Read the model definition and answer for the solid it produces. Units are mm, in the model's axes. Face numbers are marked on the shaded views. A direction names the side the tool comes from. Coordinates: 2 decimals unless noted, no trailing zeros. Order: outer loops, then holes, each group sorted by start corner. A loop starts at its lowest first (then second) coordinate and runs counter-clockwise, first axis right, second up. Notation, with made-up numbers: (19, -28) -> (30, -28) arc R13 ccw to (30, -8) -> close; hole circle Ø1 at (-24.75, 0.5). An arc over 180 degrees is marked (long way). Return JSON: item names as keys, results as strings. Group by question number.
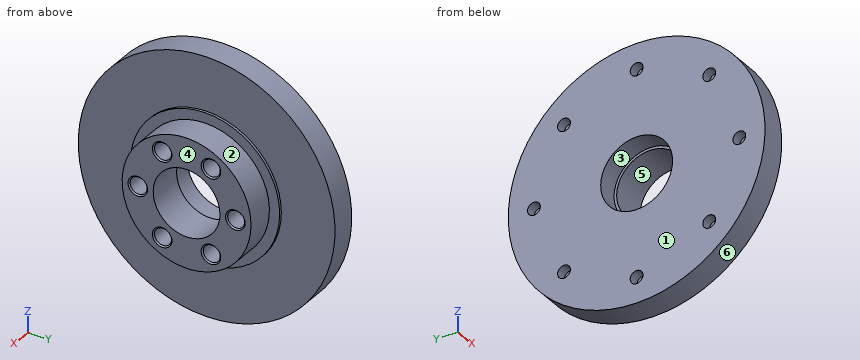
```python
from build123d import *

# Parameters (mm, degrees)
SKETCH3_R          = 2.5
CUT_EXTRUDE1_DEPTH = 4
SKETCH4_R          = 3.3
CUT_EXTRUDE2_DEPTH = 10
CHAMFER1_SIZE      = 0.5


with BuildPart() as part:
    # Sketch2 → Revolve1 (revolve)
    with BuildSketch(Plane.XY, mode=Mode.PRIVATE) as revolve1_sk:
        Polygon((0, 50), (10, 50), (10, 29.1), (11, 29.1), (11, 25.1), (22, 25.1), (22, 13), (8, 13), (8, 14), (0, 14), align=None)
    revolve(revolve1_sk.sketch.rotate(Axis((0, 0, 0), (1, 0, 0)), 90), axis=Axis((0, 0, 0), (1, 0, 0)))

    # Sketch3 → Cut-Extrude1 (cut)
    with BuildSketch(Plane(origin=(0, 0, 0), x_dir=(0, 0, -1), z_dir=(1, 0, 0))):
        with Locations((0, 40)):
            Circle(SKETCH3_R)
        with Locations((28.284271247, 28.284271247)):
            Circle(SKETCH3_R)
        with Locations((40, 0)):
            Circle(SKETCH3_R)
        with Locations((28.284271247, -28.284271247)):
            Circle(SKETCH3_R)
        with Locations((0, -40)):
            Circle(SKETCH3_R)
        with Locations((-28.284271247, -28.284271247)):
            Circle(SKETCH3_R)
        with Locations((-40, 0)):
            Circle(SKETCH3_R)
        with Locations((-28.284271247, 28.284271247)):
            Circle(SKETCH3_R)
    extrude(amount=CUT_EXTRUDE1_DEPTH, mode=Mode.SUBTRACT)

    # Sketch4 → Cut-Extrude2 (cut)
    with BuildSketch(Plane(origin=(22, 0, 0), x_dir=(0, 0, -1), z_dir=(1, 0, 0))):
        with Locations((0, 19)):
            Circle(SKETCH4_R)
        with Locations((16.454482672, 9.5)):
            Circle(SKETCH4_R)
        with Locations((16.454482672, -9.5)):
            Circle(SKETCH4_R)
        with Locations((0, -19)):
            Circle(SKETCH4_R)
        with Locations((-16.454482672, -9.5)):
            Circle(SKETCH4_R)
        with Locations((-16.454482672, 9.5)):
            Circle(SKETCH4_R)
    extrude(amount=-CUT_EXTRUDE2_DEPTH, mode=Mode.SUBTRACT)

    # Chamfer1
    chamfer1_edges = [part.edges().sort_by_distance(p)[0] for p in [
        (22, 19, 3.3),
        (22, 9.5, 19.754482672),
        (22, -9.5, 19.754482672),
        (22, -19, 3.3),
        (22, -9.5, -13.154482672),
        (22, 9.5, -13.154482672),
    ]]
    chamfer(chamfer1_edges, length=CHAMFER1_SIZE)


solid = part.part
```
1. Find section D-D on x = 2. Give the number of separate pieces and of enclosed holes in the cut face, and give its area (3 significant figures).
2. Find section A-A on x = 13.5. Determine the outline of the cut face in (y, z).
3. Which of the six approach directions +Z, -Z, +X, -X, +Y, -Y give full straight-line access (tool end or side, diameter ignored) to the marked faces 1 and 2?
4. Given pin 1 (3 mm diameter, centred on y = 0, z = 40, fed in from -X); pin 2 (8 mm diameter, centred on y = 28.28, z = 28.28, fed in from +X); pin 3 (12 mm diameter, centred on x = 19.5, z = -18, fed in from -Y), each flat-ended and moving along its own axis, determine where each tip first touches the part or whether it passes through.
5. Find section C-C on z = 40. Determine the outline of the cut face in (x, y), and give its area (3 significant figures).
6. Straight lines are drawn through the part: L1, parallel to Y at x = 15, z = 0; L2, parallel to Y at x = 3.05, z = 0; L3, parallel to X at y = 16, z = -38. For each, find the intervals that lie inside material, in ascending order.
7. Find section B-B on y = 0. Determine the outline of the cut face in (x, z), and give its area (3 significant figures).
8. For a pull along Y with two mould halves and no side action, classify the marked faces 3, 4, 5 and 6 as released by +Y, released by -Y, zero draft, split by the parting line, or undercut.
Result:
{
 "1": {"separate pieces": "1", "enclosed holes": "9", "area": "7,080 mm^2"},
 "2": {"outline": "circle Ø50.2 at (0, 0); hole circle Ø6.6 at (-19, 0); hole circle Ø26 at (0, 0); hole circle Ø6.6 at (-9.5, -16.45); hole circle Ø6.6 at (-9.5, 16.45); hole circle Ø6.6 at (9.5, -16.45); hole circle Ø6.6 at (9.5, 16.45); hole circle Ø6.6 at (19, 0)"},
 "3": {"face 1": "+Z, -Z, -X, +Y, -Y", "face 2": "+X"},
 "4": {"pin 1": "x = 4", "pin 2": "x = 10", "pin 3": "y = -22.05"},
 "5": {"outline": "(0, -30) -> (10, -30) -> (10, 30) -> (0, 30) -> (0, 2.5) -> (4, 2.5) -> (4, -2.5) -> (0, -2.5) -> close", "area": "580 mm^2"},
 "6": {"L1": "-25.1 to -22.3, -15.7 to -13, 13 to 15.7, 22.3 to 25.1", "L2": "-50 to -42.5, -37.5 to -14, 14 to 37.5, 42.5 to 50", "L3": "0 to 10"},
 "7": {"outline": "(0, -50) -> (10, -50) -> (10, -29.1) -> (11, -29.1) -> (11, -25.1) -> (22, -25.1) -> (22, -13) -> (8, -13) -> (8, -14) -> (0, -14) -> (0, -37.5) -> (4, -37.5) -> (4, -42.5) -> (0, -42.5) -> close; (0, 14) -> (8, 14) -> (8, 13) -> (22, 13) -> (22, 25.1) -> (11, 25.1) -> (11, 29.1) -> (10, 29.1) -> (10, 50) -> (0, 50) -> (0, 42.5) -> (4, 42.5) -> (4, 37.5) -> (0, 37.5) -> close", "area": "982 mm^2"},
 "8": {"face 3": "undercut", "face 4": "zero draft", "face 5": "undercut", "face 6": "split by the parting line"}
}
